Autodesk Fusion 360 part; units mm, degrees
sketch "Sketch1" plane through (0, 0, 0) normal (0, 0, 1) x (1, 0, 0)
  line L0 (17, 118.5) -> (-17, 118.5)
  line L1 (-17, 118.5) -> (-17, -118.5)
  line L2 (-17, -118.5) -> (17, -118.5)
  line L3 (17, -118.5) -> (17, 118.5)
  line L4 (17, 118.5) -> (12, 118.5)
  line L5 (12, 118.5) -> (12, 110.5) construction
  line L6 (12, 110.5) -> (17, 110.5) construction
  line L7 (17, 110.5) -> (17, 118.5)
  line L8 (-17, 118.5) -> (-12, 118.5)
  line L9 (-12, 118.5) -> (-12, 110.5) construction
  line L10 (-12, 110.5) -> (-17, 110.5) construction
  line L11 (-17, 110.5) -> (-17, 118.5)
  line L12 (-17, -118.5) -> (-12, -118.5)
  line L13 (-12, -118.5) -> (-12, -110.5) construction
  line L14 (-12, -110.5) -> (-17, -110.5) construction
  line L15 (-17, -110.5) -> (-17, -118.5)
  line L16 (17, -118.5) -> (12, -118.5)
  line L17 (12, -118.5) -> (12, -110.5) construction
  line L18 (12, -110.5) -> (17, -110.5) construction
  line L19 (17, -110.5) -> (17, -118.5)
  line L20 (12, 110.5) -> (12, 68.5) construction
  line L21 (-12, 110.5) -> (-12, 68.5) construction
  line L22 (12, -110.5) -> (12, -68.5) construction
  line L23 (-12, -110.5) -> (-12, -68.5) construction
  circle A0 centre (-12, -68.5) radius 2
  circle A1 centre (12, -68.5) radius 2
  circle A2 centre (12, -110.5) radius 2
  circle A3 centre (-12, -110.5) radius 2
  circle A4 centre (-12, 110.5) radius 2
  circle A5 centre (12, 110.5) radius 2
  dimension "d3" = 34
  dimension "d4" = 237
  dimension "d5" = 5
  dimension "d6" = 8
  dimension "d7" = 5
  dimension "d8" = 8
  dimension "d9" = 5
  dimension "d10" = 8
  dimension "d11" = 5
  dimension "d12" = 8
  dimension "d13" = 42
  dimension "d14" = 42
  dimension "d15" = 42
  dimension "d16" = 42
  dimension "d17" = 4
  dimension "d18" = 4
  dimension "d19" = 4
  dimension "d20" = 4
  dimension "d21" = 4
  dimension "d22" = 4
extrude "Extrude1" add sketch "Sketch1" along normal blind 4
The model under review builds one solid part; all positions refer to its coordinate system, in mm. Round coordinates to 2 decimals unless told otherwise and drop trailing zeros. Order: outer loops, then holes, each group sorted by start corner. A loop starts at its lowest first (then second) coordinate and runs counter-clockwise, first axis right, second up.
(1) Wall thickness on L1, parallel to Y at x = 12, z = 1.2: over which ranges is the line inside the solid? List them lowest first.
Working result:
L1: y = -118.5 to -112.5, -108.5 to -70.5, -66.5 to 108.5, 112.5 to 118.5
(2) For P1, Ø2.5, axis at x = -12, y = -110.5, coming from the +Z side, flat-tipped, find the tip position at first contact; note if it passes through.
Working result:
P1: passes through
(3) Take a section at B-B, the plane x = -12. State the section outline as (y, z) points, plus the area to 3 significant figures.
Working result:
outline: (-118.5, 0) - (-112.5, 0) - (-112.5, 4) - (-118.5, 4) - close; (-108.5, 0) - (-70.5, 0) - (-70.5, 4) - (-108.5, 4) - close; (-66.5, 0) - (108.5, 0) - (108.5, 4) - (-66.5, 4) - close; (112.5, 0) - (118.5, 0) - (118.5, 4) - (112.5, 4) - close
area: 900 mm2
(4) Take a section at A-A, the plane y = -68.5. State the section outline as (x, z) points, plus the area to 3 significant figures.
Working result:
outline: (-17, 0) - (-14, 0) - (-14, 4) - (-17, 4) - close; (-10, 0) - (10, 0) - (10, 4) - (-10, 4) - close; (14, 0) - (17, 0) - (17, 4) - (14, 4) - close
area: 104 mm2
(5) Mouldability with a two-part tool opening along X and no side actions: class faces 1 (the face through (0, 2, 4)), 2 (the face through (11.74, -112.483, 1.972)), 3 (the face through (17, -2, 2)) as released by +X, released by -X, zero draft, split by the parting line, or undercut.
Working result:
face 1: zero draft
face 2: undercut
face 3: released by +X
